For this review, use the dimensioned drawing (mm, ordinates from the lowest corner) and the shaded views. Round coordinates to 2 decimals unless told otherwise and drop trailing zeros. Order: outer loops, then holes, each group sorted by start corner. A loop starts at its lowest first (then second) coordinate and runs counter-clockwise, first axis right, second up. Notation, with made-up numbers: (0, 24.25) - (19, 24.25) arc R27 cw to (19, 53.25) - close; hole circle Ø7 at (87.25, 73). An arc over 180 degrees is marked (long way). Write item = value, one per line.
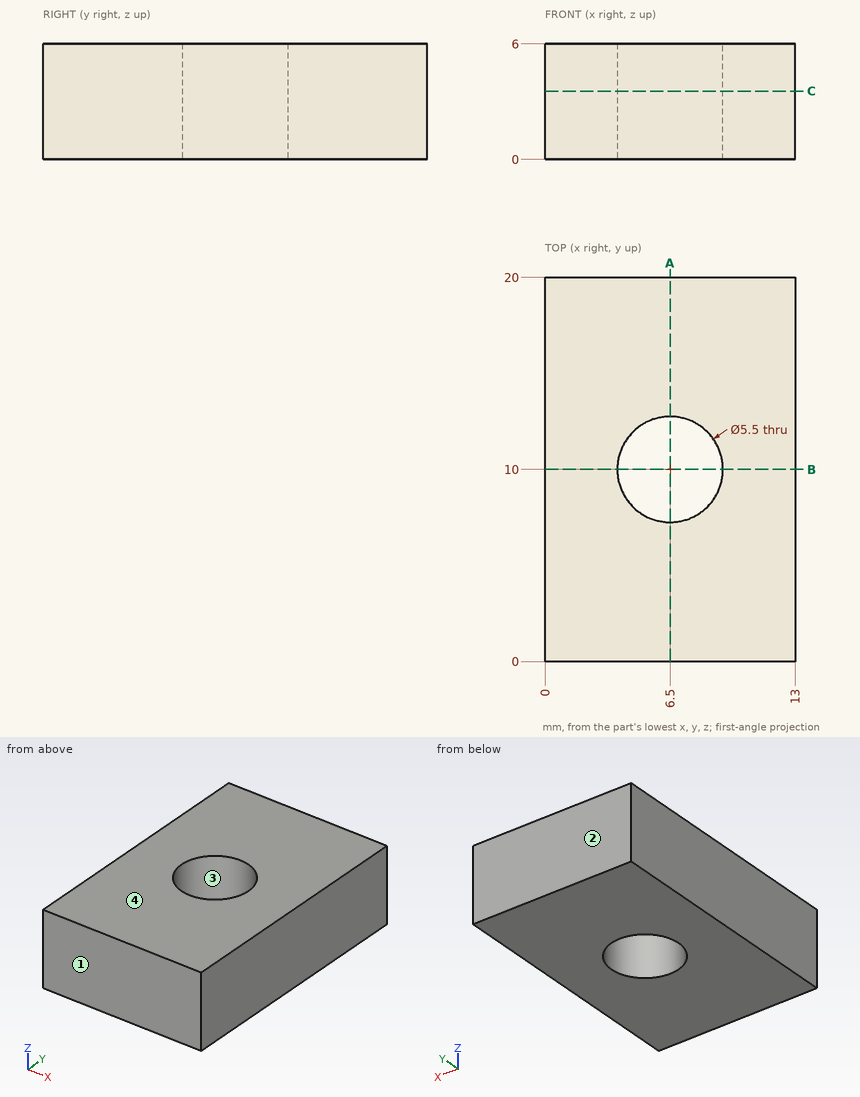
Item 1: For line 1 along Y through (x, z) = (6.5, 1.75); line 2 along X through (y, z) = (9.5, 3.65); line 3 along Y through (x, z) = (5, 3.9), list the stretches that pass through material, from the lowest coordinate up. Write a range as [from, to].
Data:
line_1 = [0, 7.25], [12.75, 20]
line_2 = [0, 3.8], [9.2, 13]
line_3 = [0, 7.7], [12.3, 20]
Item 2: Insertion check: P1, Ø4.5, axis at x = 6.5, y = 10, coming from the +Z side. The pin has a flat end and moves straight along its axis. Give the tip position at first contact, or say it passes through.
Data:
P1 = through
Item 3: The part is to be moulded in two halves that separate along Y. For the marked faces 1, 2, 3 and 4, say which applies: +Y half, -Y half, draft (parallel to the pull), parting line (faces both ways), or undercut.
Data:
face_1 = -Y half
face_2 = +Y half
face_3 = undercut
face_4 = draft
Item 4: Take a section at A-A, the plane x = 6.5. State the section outline as (y, z) points, and give its area (3 significant figures).
Data:
outline = (0, 0) - (7.25, 0) - (7.25, 6) - (0, 6) - close; (12.75, 0) - (20, 0) - (20, 6) - (12.75, 6) - close
area = 87.0 mm2
Item 5: Take a section at B-B, the plane y = 10. State the section outline as (x, z) points.
Data:
outline = (0, 0) - (3.75, 0) - (3.75, 6) - (0, 6) - close; (9.25, 0) - (13, 0) - (13, 6) - (9.25, 6) - close
Item 6: Take a section at C-C, the plane z = 3.55. State the section outline as (x, y) points.
Data:
outline = (0, 0) - (13, 0) - (13, 20) - (0, 20) - close; hole circle Ø5.5 at (6.5, 10)
